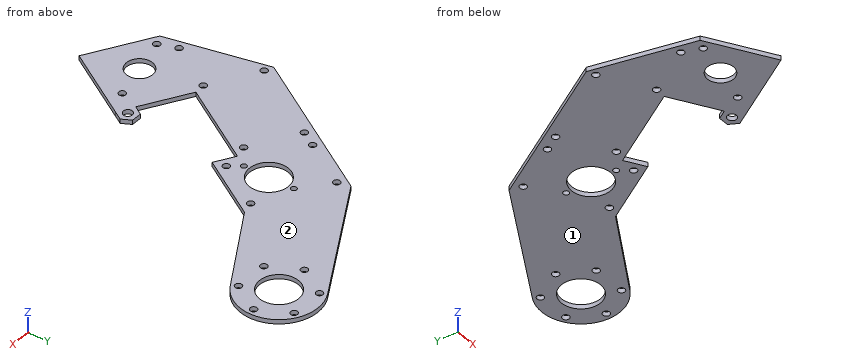
from build123d import *

# Parameters (mm, degrees)
SKETCH1_R                   = 14.2875
SKETCH1_R_2                 = 9.525
BOSS_EXTRUDE1_DEPTH         = 3.175
F_10_CLEARANCE_HOLE2_D      = 4.9784
F_10_CLEARANCE_HOLE3_D      = 4.9784
F_1_4_CLEARANCE_HOLE1_D     = 6.5278
F_20_0_161_DIAMETER_HOLE1_D = 4.0894


with BuildPart() as part:
    # Sketch1 → Boss-Extrude1 (new body)
    with BuildSketch(Plane.XY.offset(-14.194599474)):
        with BuildLine():
            Line((-11.403602879, 461.040918113), (18.881283072, 509.506866808))
            Line((18.881283072, 509.506866808), (22.784668372, 515.753589084))
            Line((22.784668372, 515.753589084), (19.342339301, 522.227668471))
            Line((19.342339301, 522.227668471), (12.014457551, 522.48356374))
            Line((12.014457551, 522.48356374), (8.11107225, 516.236841464))
            Line((8.11107225, 516.236841464), (-23.846467356, 536.206128526))
            Line((-23.846467356, 536.206128526), (10.759214603, 591.586796266))
            Line((10.759214603, 591.586796266), (24.22197813, 583.174327946))
            Line((24.22197813, 583.174327946), (51.141876753, 626.255171231))
            Line((51.141876753, 626.255171231), (112.462044501, 660.93728694))
            ThreePointArc((112.462044501, 660.93728694), (123.365099157, 699.702028841), (84.677956887, 710.877306848))
            Line((84.677956887, 710.877306848), (-5.401730059, 661.587538174))
            Line((-5.401730059, 661.587538174), (-69.615486106, 558.824047132))
            Line((-69.615486106, 558.824047132), (-54.307899735, 487.850498283))
            Line((-54.307899735, 487.850498283), (-11.403602879, 461.040918113))
        make_face()
        with Locations((16.14150623, 618.174698631)):
            Circle(SKETCH1_R, mode=Mode.SUBTRACT)
        with Locations((-22.373657227, 496.622766323)):
            Circle(SKETCH1_R_2, mode=Mode.SUBTRACT)
        with Locations((98.394472266, 685.809641802)):
            Circle(SKETCH1_R, mode=Mode.SUBTRACT)
    extrude(amount=BOSS_EXTRUDE1_DEPTH)

    # #10 Clearance Hole2 (through all)
    with Locations(Plane.XY.offset(-11.019599474)):
        with Locations((2.375342418, 502.336523103), (-47.122656873, 490.909009542), (-3.381611976, 652.837445435), (42.391784014, 624.235053148), (22.201860047, 591.924420685), (-23.571535943, 620.526812972), (-31.474844299, 535.981130963), (-63.785476762, 556.17105493), (-51.664768266, 503.670498499), (2.009121865, 589.566678183), (-30.301510599, 609.756602151)):
            Hole(F_10_CLEARANCE_HOLE2_D / 2)

    # #10 Clearance Hole3 (through all)
    with Locations(Plane.XY.offset(-11.019599474)):
        with Locations((111.013174745, 706.003787092), (122.192466334, 684.978597537), (109.573763855, 664.784452247), (85.775769786, 665.615496512), (74.596478197, 686.640686067), (87.215180677, 706.834831357)):
            Hole(F_10_CLEARANCE_HOLE3_D / 2)

    # 1/4 Clearance Hole1 (through all)
    with Locations(Plane.XY.offset(-11.019599474)):
        with Locations((15.456786622, 516.009484354)):
            Hole(F_1_4_CLEARANCE_HOLE1_D / 2)

    # #20 (0.161) Diameter Hole1 (through all)
    with Locations(Plane(origin=(0, 0, -14.194599474), x_dir=(-1, 0, 0), z_dir=(0, 0, -1))):
        with Locations((-16.141506225, 636.208698631), (-16.141506234, 600.140698631)):
            Hole(F_20_0_161_DIAMETER_HOLE1_D / 2)


solid = part.part
Here's how the part is built. I have some questions about the finished solid (model axes, mm). Face numbers are marked on the shaded views. Round coordinates to 2 decimals unless told otherwise and drop trailing zeros. Loops run counter-clockwise (first coordinate to the right, second up) from the corner with the lowest first, then second, coordinate; pieces in that order, holes last.
1. If we section it at C-C on z = -13.4: Count the separate pieces of the cut face and the enclosed holes in it, plus the area to 3 significant figures.
Answer list:
separate pieces: 1
enclosed holes: 23
area: 15,600 mm2
2. If I drill on line 1 along Y through (x, z) = (-22, -13.85); line 2 along X through (y, z) = (626.5, -11.2); line 3 along X through (y, z) = (665.5, -12.4), over which ranges is the centre line in solid material (lowest first)?
Answer list:
line 1: y = 467.66 to 487.11, 506.14 to 535.05, 539.16 to 618.6, 622.46 to 635.02
line 2: x = -27.33 to 4.53, 27.75 to 41.36, 43.42 to 51.57
line 3: x = 1.75 to 83.29, 88.26 to 107.19, 111.96 to 118.5
3. If we section it at D-D on x = 63: Write out the boundary of the cut face in (y, z).
Answer list:
outline: (632.96, -14.19) - (699.02, -14.19) - (699.02, -11.02) - (632.96, -11.02) - close
4. For P1, Ø6.5, axis at x = 22.2, y = 591.92, coming from the -Z side; P2, Ø1, axis at x = 81.5, z = -13, coming from the -Y side; P3, Ø1.5, axis at x = 47, z = -11.5, coming from the -Y side; P4, Ø1, axis at y = 634.5, z = -13, coming from the -X side, each with a flat end and sliding along its axis, tell me the tip position at first contact or that it passes through.
Answer list:
P1: stops at z = -14.19
P2: stops at y = 643.14
P3: stops at y = 618.43
P4: stops at x = -22.64
5. If we section it at A-A on x = -17: Write out the boundary of the cut face in (y, z), plus the area to 3 significant figures.
Answer list:
outline: (464.54, -14.19) - (488.76, -14.19) - (488.76, -11.02) - (464.54, -11.02) - close; (504.49, -14.19) - (531.93, -14.19) - (531.93, -11.02) - (504.49, -11.02) - close; (547.16, -14.19) - (643.03, -14.19) - (643.03, -11.02) - (547.16, -11.02) - close
area: 468 mm2
6. We'd pull the mould along Z, two halves only. Please class the marked faces 1 and 2: +Z half, -Z half, draft (parallel to the pull), parting line (faces both ways), or undercut.
Answer list:
face 1: -Z half
face 2: +Z half
7. If we section it at B-B on x = 35: Write out the boundary of the cut face in (y, z).
Answer list:
outline: (600.42, -14.19) - (683.69, -14.19) - (683.69, -11.02) - (600.42, -11.02) - close
